Could you check a few things on this drawing? It's one solid part, dimensions in mm from its lowest x, y, z. A direction names the side the tool comes from. Give positions to 0.01 mm unless a question says otherwise; leave off trailing zeros. Order: outer loops, then holes, each group sorted by start corner. A loop starts at its lowest first (then second) coordinate and runs counter-clockwise, first axis right, second up. Notation, with made-up numbers: (48.25, -26.5) -> (57.25, -26.5) arc R9 cw to (57.25, -21.5) -> close; hole circle Ø11 at (52, 76). An arc over 180 degrees is marked (long way). Write each question's results on one line, items separated by ' | '. Start each with the question number.
Q1. Imagine slicing it at D-D, the plane z = 3.75. Please give me the cut outline in (x, y).
Q2. For the marked faces 1, 2, 3, 4 and 5, which set-ups out of +Z, -Z, +X, -X, +Y, -Y let a thin tool reach every point of the face, with its end or its side?
Q3. I need wall thicknesses on line 1 along Y through (x, z) = (14.25, 18); line 2 along X through (y, z) = (50, 12.5). Which ranges of each line are inside material? Lowest first, please. Write a range as [from, to].
Q4. Imagine slicing it at B-B, the plane z = 11. Please give me the cut outline in (x, y), then the cut area to 3 significant figures.
Q5. I'm going to push flat-ended pins straight in: pin 1 (8 mm diameter, centred on x = 9, y = 45.5, fed in from -Z); pin 2 (5 mm diameter, centred on x = 7.5, z = 15, fed in from -Y); pin 3 (2 mm diameter, centred on y = 76.5, z = 15.5, fed in from -X); pin 4 (1.8 mm diameter, centred on y = 45.5, z = 11, fed in from -X). Where does each tip first touch, or does it pass through?
Q6. Imagine slicing it at A-A, the plane x = 8.25. Please give me the cut outline in (y, z).
Q7. Imagine slicing it at C-C, the plane y = 33.5. Please give me the cut outline in (x, z).
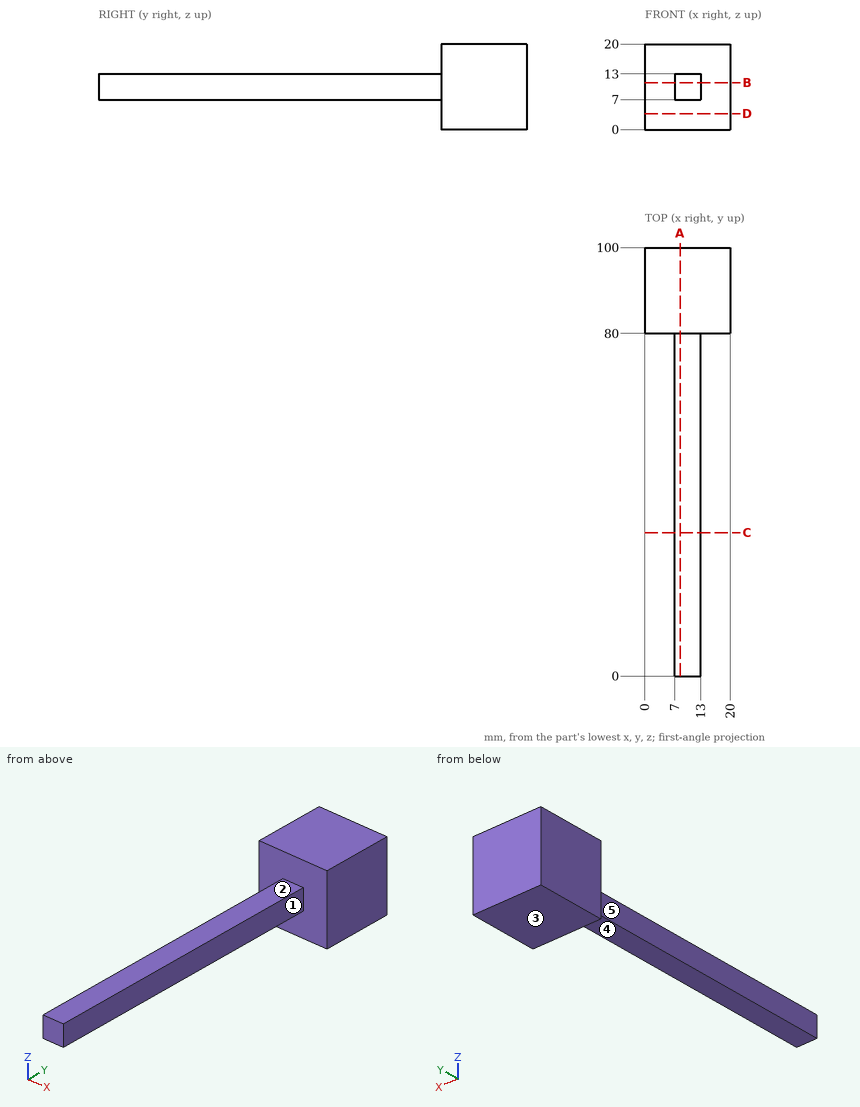
Geometry check:
1) outline: (0, 80) -> (20, 80) -> (20, 100) -> (0, 100) -> close
2) face 1: +Z, -Z, +X, -Y | face 2: +Z, +X, -X, -Y | face 3: -Z, +X, -X, +Y, -Y | face 4: -Z, +X, -X, -Y | face 5: +Z, -Z, -X, -Y
3) line 1: [80, 100] | line 2: [7, 13]
4) outline: (0, 80) -> (7, 80) -> (7, 0) -> (13, 0) -> (13, 80) -> (20, 80) -> (20, 100) -> (0, 100) -> close | area: 880 mm²
5) pin 1: z = 7 | pin 2: y = 0 | pin 3: through | pin 4: x = 7
6) outline: (0, 7) -> (80, 7) -> (80, 0) -> (100, 0) -> (100, 20) -> (80, 20) -> (80, 13) -> (0, 13) -> close
7) outline: (7, 7) -> (13, 7) -> (13, 13) -> (7, 13) -> close
